Input: part model. Units: mm. Frame: model coordinates. Round coordinates to 2 decimals unless told otherwise and drop trailing zeros. Write each loop counter-clockwise with the first axis right and the second up, starting at its lowest first coordinate (ties: lowest second). Pieces come first, ordered by that corner, then holes. Notation, with made-up numbers: (26.25, 37) -> (78.25, 37) arc R8 cw to (78.25, 47) -> close; hole circle Ø2 at (-37.5, 84). An arc over 180 degrees is marked (long way). Write item = value, one per line. Start each with the question number.
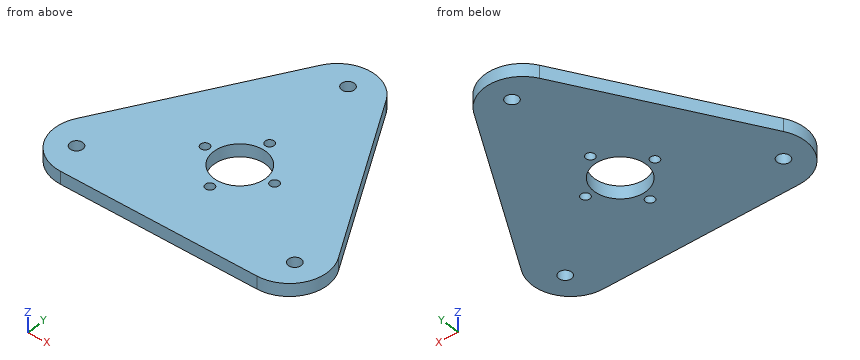
Autodesk Inventor part; units mm, degrees
ref_plane "YZ Plane" through (0, 0, 0) normal (1, 0, 0) x (0, 1, 0)
ref_plane "XZ Plane" through (0, 0, 0) normal (0, 1, 0) x (-1, 0, 0)
ref_plane "XY Plane" through (0, 0, 0) normal (0, 0, 1) x (1, 0, 0)
sketch "Sketch2" plane through (0, 0, 0) normal (0, 0, 1) x (1, 0, 0)
  circle A0 centre (0, 0) radius 3.9688
  circle A1 centre (0, 63.5) radius 3.175
  circle A2 centre (-54.9926, -31.75) radius 3.175
  circle A3 centre (54.9926, -31.75) radius 3.175
  line L0 (0, 69.85) -> (60.4919, -34.925) construction
  line L1 (60.4919, -34.925) -> (-60.4919, -34.925) construction
  line L2 (-60.4919, -34.925) -> (0, 69.85) construction
  line L3 (0, 95.25) -> (82.4889, -47.625)
  line L4 (82.4889, -47.625) -> (-82.4889, -47.625)
  line L5 (-82.4889, -47.625) -> (0, 95.25)
  circle A4 centre (0, 0) radius 17.5006 construction
  circle A5 centre (0, 17.5006) radius 2.25
  circle A6 centre (-17.5006, 0) radius 2.25
  circle A7 centre (0, -17.5006) radius 2.25
  circle A8 centre (17.5006, 0) radius 2.25
  circle A9 centre (0, 0) radius 12.954
  dimension "d14" = 35.0012
  dimension "d0" = 7.9375
  dimension "d1" = 6.35
  dimension "d2" = 63.5
  dimension "d5" = 360
  dimension "d8" = 12.7
  dimension "d9" = 12.7
  dimension "d10" = 12.7
  dimension "d15" = 4.5
  dimension "d18" = 360
  dimension "d20" = 25.908
extrude "Extrusion1" add sketch "Sketch2" along normal blind 6.35 contours L3 L4 L5
fillet "Fillet1" radius 19.05 3 edges at (0, 95.25, 3.175) (-82.4889, -47.625, 3.175) (82.4889, -47.625, 3.175)
properties part number "Triangle-motor-hole"
1. Section A-A (x = 0). Output: boundary loops of the cut face in (y, z) (3 decimals).
2. Section B-B (y = 0). Output: boundary loops of the cut face in (x, z), then the cut area to 3 significant figures.
3. Section D-D (z = 5). State how many separate pieces and enclosed holes the cut face has, then the cut area to 3 significant figures.
4. Line query: line 1 along Y through (x, z) = (0, 5) (3 decimals); line 2 along X through (y, z) = (17.5, 2.25); line 3 along Y through (x, z) = (-18, 1) (3 decimals). Output: solid intervals per line, ascending.
5. Section C-C (y = -31.75). Output: boundary loops of the cut face in (x, z).
6. Pin query (flat end, axial travel): P1, Ø2, axis at x = 49.5, z = 1, coming from the +Y side; P2, Ø5, axis at x = 0, y = -17.5, coming from the -Z side; P3, Ø3, axis at y = 41.5, z = 4, coming from the -X side; P4, Ø1, axis at y = 53.5, z = 4.5, coming from the +X side. Return the tip coordinate at first contact, or that it passes through.
Check sheet entries:
q1.outline = (-47.625, 0) -> (-19.751, 0) -> (-19.751, 6.35) -> (-47.625, 6.35) -> close; (-15.251, 0) -> (-12.954, 0) -> (-12.954, 6.35) -> (-15.251, 6.35) -> close; (12.954, 0) -> (15.251, 0) -> (15.251, 6.35) -> (12.954, 6.35) -> close; (19.751, 0) -> (60.325, 0) -> (60.325, 6.35) -> (19.751, 6.35) -> close; (66.675, 0) -> (76.2, 0) -> (76.2, 6.35) -> (66.675, 6.35) -> close
q2.outline = (-54.99, 0) -> (-19.75, 0) -> (-19.75, 6.35) -> (-54.99, 6.35) -> close; (-15.25, 0) -> (-12.95, 0) -> (-12.95, 6.35) -> (-15.25, 6.35) -> close; (12.95, 0) -> (15.25, 0) -> (15.25, 6.35) -> (12.95, 6.35) -> close; (19.75, 0) -> (54.99, 0) -> (54.99, 6.35) -> (19.75, 6.35) -> close
q2.area = 477 mm2
q3.separate_pieces = 1
q3.enclosed_holes = 8
q3.area = 10,400 mm2
q4.line_1 = -47.625 to -19.751, -15.251 to -12.954, 12.954 to 15.251, 19.751 to 60.325, 66.675 to 76.2
q4.line_2 = -44.89 to -2.25, 2.25 to 44.89
q4.line_3 = -47.625 to -2.194, 2.194 to 64.073
q5.outline = (-68.28, 0) -> (-58.17, 0) -> (-58.17, 6.35) -> (-68.28, 6.35) -> close; (-51.82, 0) -> (51.82, 0) -> (51.82, 6.35) -> (-51.82, 6.35) -> close; (58.17, 0) -> (68.28, 0) -> (68.28, 6.35) -> (58.17, 6.35) -> close
q6.P1 = 11.25
q6.P2 = 0
q6.P3 = -31.9
q6.P4 = 24.39
